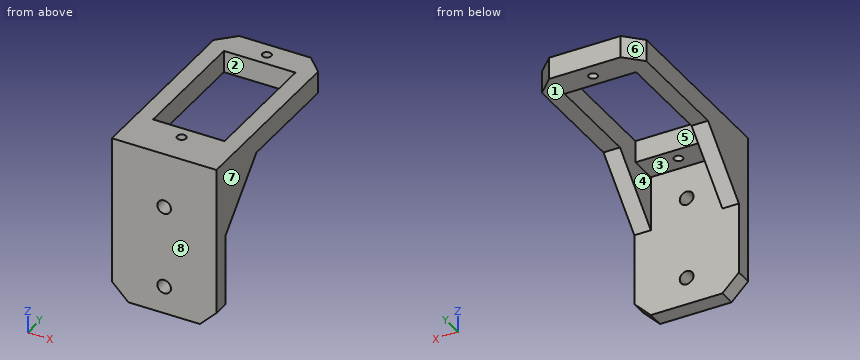
from build123d import *

# Parameters (mm, degrees)
CROQUIS1_W              = 19
CROQUIS1_H              = 33
SALIENTE_EXTRUIR1_DEPTH = 4
CROQUIS2_R              = 0.8
CROQUIS2_W              = 13
CROQUIS2_H              = 23
CORTAR_EXTRUIR1_DEPTH   = 5
CHAFL_N1_SIZE           = 3
CROQUIS3_W              = 19
CROQUIS3_H              = 3
SALIENTE_EXTRUIR2_DEPTH = 30
SALIENTE_EXTRUIR3_DEPTH = 3
SALIENTE_EXTRUIR4_DEPTH = 3
CHAFL_N2_SIZE           = 3
CROQUIS9_R              = 1.25
CORTAR_EXTRUIR2_DEPTH   = 3


with BuildPart() as part:
    # Croquis1 → Saliente-Extruir1 (new body)
    with BuildSketch(Plane.XY):
        Rectangle(CROQUIS1_W, CROQUIS1_H)
    extrude(amount=SALIENTE_EXTRUIR1_DEPTH)

    # Croquis2 → Cortar-Extruir1 (cut)
    with BuildSketch(Plane.XY.offset(4)):
        with Locations((0, 13.83)):
            Circle(CROQUIS2_R)
        with Locations((0, -13.83)):
            Circle(CROQUIS2_R)
        Rectangle(CROQUIS2_W, CROQUIS2_H)
    extrude(amount=-CORTAR_EXTRUIR1_DEPTH, mode=Mode.SUBTRACT)

    # Chaflán1
    chafl_n1_edges = [part.edges().sort_by_distance(p)[0] for p in [
        (-9.5, 16.5, 2),
        (9.5, 16.5, 2),
    ]]
    chamfer(chafl_n1_edges, length=CHAFL_N1_SIZE)

    # Croquis3 → Saliente-Extruir2 (add)
    with BuildSketch(Plane.XY.offset(4)):
        with Locations((0, -18)):
            Rectangle(CROQUIS3_W, CROQUIS3_H)
    extrude(amount=-SALIENTE_EXTRUIR2_DEPTH)

    # Croquis7 → Saliente-Extruir3 (add)
    with BuildSketch(Plane(origin=(9.5, 0, 0), x_dir=(0, 0, -1), z_dir=(1, 0, 0))):
        Polygon((0, -6.5), (0, -16.5), (10, -16.5), align=None)
    extrude(amount=-SALIENTE_EXTRUIR3_DEPTH)

    # Croquis8 → Saliente-Extruir4 (add)
    with BuildSketch(Plane.ZY.offset(9.5)):
        Polygon((0, -16.5), (-10, -16.5), (0, -6.5), align=None)
    extrude(amount=-SALIENTE_EXTRUIR4_DEPTH)

    # Chaflán2
    chafl_n2_edges = [part.edges().sort_by_distance(p)[0] for p in [
        (-9.5, -18, -26),
        (9.5, -18, -26),
    ]]
    chamfer(chafl_n2_edges, length=CHAFL_N2_SIZE)

    # Croquis9 → Cortar-Extruir2 (cut)
    with BuildSketch(Plane(origin=(0, -16.5, 0), x_dir=(1, 0, 0), z_dir=(0, 1, 0))):
        with Locations((0, 6)):
            Circle(CROQUIS9_R)
        with Locations((0, 21)):
            Circle(CROQUIS9_R)
    extrude(amount=-CORTAR_EXTRUIR2_DEPTH, mode=Mode.SUBTRACT)


solid = part.part
Geometry: final body of the model. Coordinates: model frame, mm. Face numbers are marked on the shaded views. A direction names the side the tool comes from. Coordinates: 2 decimals unless noted, no trailing zeros. Loops run counter-clockwise (first coordinate to the right, second up) from the corner with the lowest first, then second, coordinate; pieces in that order, holes last. Notation, with made-up numbers: (-29.5, -2.5) - (-24.5, -2.5) arc R20 ccw to (-24.5, 16.5) - close; hole circle Ø9 at (50.5, 45). An arc over 180 degrees is marked (long way). Put each result on its own line as item: value. Start each with the question number.
Q1. Set-up query: the marked faces 1, 2, 3 and 4. Return all of +Z, -Z, +X, -X, +Y, -Y with unobstructed straight access to the full face (end or side cutting, diameter ignored); none if empty.
Q2. Cut plane C-C, the plane x = -1.75. Return loops of the section in (y, z), and give its area (3 significant figures).
Q3. Cut plane A-A, the plane y = 6.5. Return loops of the section in (x, z).
Q4. Cut plane B-B, the plane z = -21. Return loops of the section in (x, y), and give its area (3 significant figures).
Q5. Pull-direction query (Y, two-part tool) for the marked faces 5, 6, 7 and 8; classes: released by +Y, released by -Y, zero draft, split by the parting line, or undercut.
Q6. Line query: line 1 (Z direction, x = 0, y = -17.2); line 2 (Y direction, x = 0, z = 2.9); line 3 (X direction, y = -14, z = -1). Output: solid intervals per line, ascending.
Q7. Cut plane D-D, the plane z = 1. Return loops of the section in (x, y), and give its area (3 significant figures).
Q8. Pin query (flat end, axial travel): pin 1 Ø1.8 at (x, y) = (0, 13.83) entering from -Z; pin 2 Ø4 at (x, z) = (0, -6) entering from +Y. Return the tip coordinate at first contact, or that it passes through.
Filled sheet:
1. face 1: -Z, +X, -X, +Y
1. face 2: +Z, -Z
1. face 3: -Z, +Y
1. face 4: -Z
2. outline: (-19.5, -26) - (-16.5, -26) - (-16.5, 0) - (-11.5, 0) - (-11.5, 4) - (-19.5, 4) - close; (11.5, 0) - (16.5, 0) - (16.5, 4) - (11.5, 4) - close
2. area: 130 mm²
3. outline: (-9.5, 0) - (-6.5, 0) - (-6.5, 4) - (-9.5, 4) - close; (6.5, 0) - (9.5, 0) - (9.5, 4) - (6.5, 4) - close
4. outline: (-9.5, -19.5) - (-1.25, -19.5) - (-1.25, -16.5) - (-9.5, -16.5) - close; (1.25, -19.5) - (9.5, -19.5) - (9.5, -16.5) - (1.25, -16.5) - close
4. area: 49.5 mm²
5. face 5: undercut
5. face 6: released by +Y
5. face 7: zero draft
5. face 8: released by -Y
6. line 1: -26 to -22.25, -19.75 to -7.25, -4.75 to 4
6. line 2: -19.5 to -14.63, -13.03 to -11.5, 11.5 to 13.03, 14.63 to 16.5
6. line 3: -9.5 to -6.5, 6.5 to 9.5
7. outline: (-9.5, -19.5) - (9.5, -19.5) - (9.5, 13.5) - (6.5, 16.5) - (-6.5, 16.5) - (-9.5, 13.5) - close; hole (-6.5, -11.5) - (6.5, -11.5) - (6.5, 11.5) - (-6.5, 11.5) - close; hole circle Ø1.6 at (0, -13.83); hole circle Ø1.6 at (0, 13.83)
7. area: 372 mm²
8. pin 1: z = 0
8. pin 2: y = -16.5
